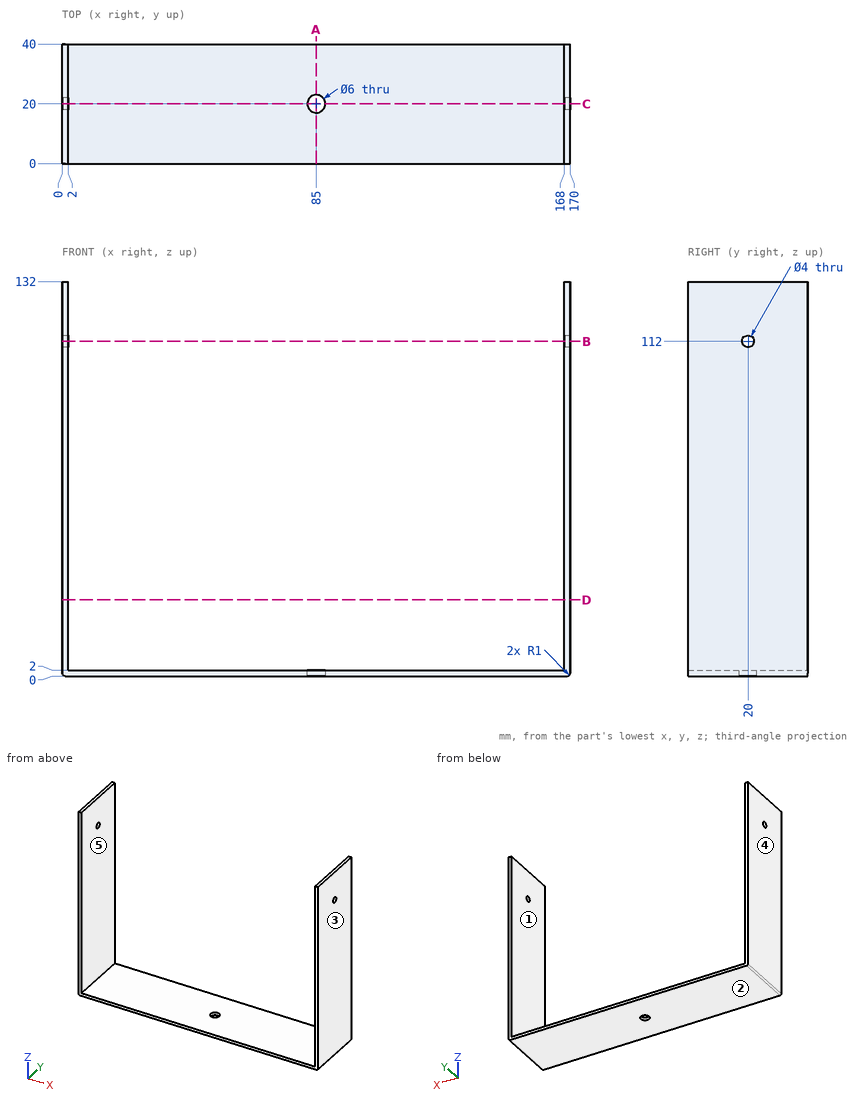
Input: dimensioned drawing with shaded views. Units: mm. Origin: part minimum x, y, z. A direction names the side the tool comes from. Give positions to 0.01 mm unless a question says otherwise; leave off trailing zeros. Loops run counter-clockwise (first coordinate to the right, second up) from the corner with the lowest first, then second, coordinate; pieces in that order, holes last. Notation, with made-up numbers: (29.25, -16.75) -> (68.25, -16.75) arc R23 cw to (68.25, -8.75) -> close; hole circle Ø3 at (18.5, 72). An arc over 180 degrees is marked (long way). Use a Markdown table: item, result. Add a question column.
1) Section query C-C, the plane y = 20. Return the cut outline in (x, z).
2) Section query A-A, the plane x = 85. Return the cut outline in (y, z), then the cut area to 3 significant figures.
3) First-contact query: pin 1 (12 mm diameter, centred on x = 39, y = 12.5, fed in from +Z); pin 2 (3.5 mm diameter, centred on y = 20, z = 112, fed in from -X). Flat tips, straight axial feed; report the tip coordinate or a pass-through.
4) Pull-direction query (X, two-part tool) for the marked faces 1, 2 and 3; classes: +X half, -X half, draft (parallel to the pull), parting line (faces both ways), or undercut.
5) Line query: line 1 along X through (y, z) = (16.5, 32); line 2 along Y through (x, z) = (1.5, 112); line 3 along Y through (x, z) = (85, 1). Output: solid intervals per line, ascending. Write a range as [from, to].
6) Section query D-D, the plane z = 25.5. Return the cut outline in (x, y).
7) Reachability of the marked faces 4 and 5 from +Z, -Z, +X, -X, +Y, -Y: full face, straight path, thin tool, end or side. Return the list, or none.
8) Section query B-B, the plane z = 112. Return the cut outline in (x, y), then the cut area to 3 significant figures.
Numbers:
| question | item | result |
|---|---|---|
| 1 | outline | (0, 1) arc R1 ccw to (1, 0) -> (82, 0) -> (82, 2) -> (2, 2) -> (2, 110) -> (0, 110) -> close; (0, 114) -> (2, 114) -> (2, 132) -> (0, 132) -> close; (88, 0) -> (169, 0) arc R1 ccw to (170, 1) -> (170, 110) -> (168, 110) -> (168, 2) -> (88, 2) -> close; (168, 114) -> (170, 114) -> (170, 132) -> (168, 132) -> close |
| 2 | outline | (0, 0) -> (17, 0) -> (17, 2) -> (0, 2) -> close; (23, 0) -> (40, 0) -> (40, 2) -> (23, 2) -> close |
| 2 | area | 68.0 mm2 |
| 3 | pin 1 | stops at z = 2 |
| 3 | pin 2 | passes through |
| 4 | face 1 | undercut |
| 4 | face 2 | draft |
| 4 | face 3 | +X half |
| 5 | line 1 | x = [0, 2], [168, 170] |
| 5 | line 2 | y = [0, 18], [22, 40] |
| 5 | line 3 | y = [0, 17], [23, 40] |
| 6 | outline | (0, 0) -> (2, 0) -> (2, 40) -> (0, 40) -> close; (168, 0) -> (170, 0) -> (170, 40) -> (168, 40) -> close |
| 7 | face 4 | +Z, -Z, -X, +Y, -Y |
| 7 | face 5 | +Z, +Y, -Y |
| 8 | outline | (0, 0) -> (2, 0) -> (2, 18) -> (0, 18) -> close; (0, 22) -> (2, 22) -> (2, 40) -> (0, 40) -> close; (168, 0) -> (170, 0) -> (170, 18) -> (168, 18) -> close; (168, 22) -> (170, 22) -> (170, 40) -> (168, 40) -> close |
| 8 | area | 144 mm2 |
